Design review of the part built by this model. Coordinates are the model's own, in mm. Face numbers are marked on the shaded views. Coordinates: 2 decimals unless noted, no trailing zeros. Write each loop counter-clockwise with the first axis right and the second up, starting at its lowest first coordinate (ties: lowest second). Pieces come first, ordered by that corner, then holes.
Q1. For pin 1 Ø3 at (x, y) = (-7, 2.5) entering from +Z; pin 2 Ø4 at (x, z) = (1.5, -2.5) entering from -Y; pin 3 Ø4 at (x, y) = (14.5, 10.5) entering from +Z, all flat-tipped, find the tip position at first contact; note any pin that passes through.
Q2. The part is to be moulded in two halves that separate along X. For the marked faces 1, 2 and 3, say which applies: released by +X, released by -X, zero draft, split by the parting line, or undercut.
Q3. For L1, parallel to Y at x = 0, z = -3.5; L2, parallel to X at y = 2.25, z = 0.75; L3, parallel to X at y = 9.5, z = 0.25, list the stretches that pass through material, from the lowest coordinate up.
Q4. Take a section at B-B, the plane x = 28.5. Write out the cut boundary in (y, z).
Q5. Take a section at C-C, the plane z = 3.25. Write out the cut boundary in (x, y).
Q6. Take a section at D-D, the plane y = 11. Write out the cut boundary in (x, z), plus the area to 3 significant figures.
Q7. Take a section at A-A, the plane y = 6. Write out the cut boundary in (x, z), plus the area to 3 significant figures.
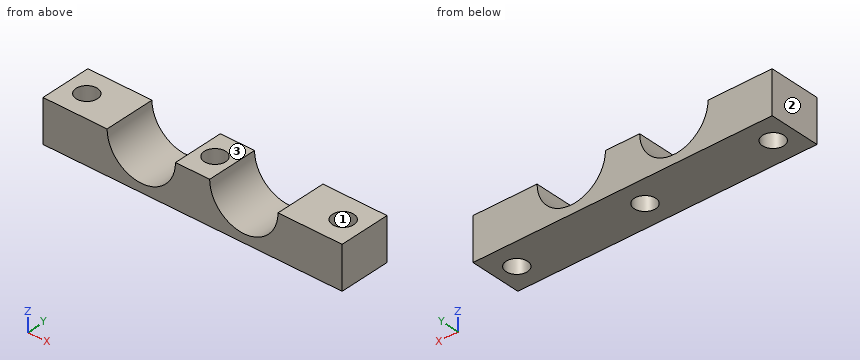
from build123d import *

# Parameters (mm, degrees)
BOSS_EXTRUDE1_DEPTH = 12
SKETCH2_R           = 2.5
CUT_EXTRUDE1_DEPTH  = 10


with BuildPart() as part:
    # Sketch1 → Boss-Extrude1 (new body)
    with BuildSketch(Plane(origin=(0, 0, 0), x_dir=(1, 0, 0), z_dir=(0, 1, 0))):
        with BuildLine():
            Line((35, 5), (-35, 5))
            Line((-35, 5), (-35, -5))
            Line((-35, -5), (-20, -5))
            ThreePointArc((-20, -5), (-12, 3), (-4, -5))
            Line((-4, -5), (4, -5))
            ThreePointArc((4, -5), (12, 3), (20, -5))
            Line((20, -5), (35, -5))
            Line((35, -5), (35, 5))
        make_face()
    extrude(amount=BOSS_EXTRUDE1_DEPTH)

    # Sketch2 → Cut-Extrude1 (cut)
    with BuildSketch(Plane(origin=(0, 0, -5), x_dir=(-1, 0, 0), z_dir=(0, 0, -1))):
        with Locations((0, 6)):
            Circle(SKETCH2_R)
        with Locations((-30, 6)):
            Circle(SKETCH2_R)
        with Locations((30, 6)):
            Circle(SKETCH2_R)
    extrude(amount=-CUT_EXTRUDE1_DEPTH, mode=Mode.SUBTRACT)


solid = part.part
Responses:
1. pin 1: stops at z = 0.34
1. pin 2: stops at y = 0
1. pin 3: stops at z = -1.61
2. face 1: undercut
2. face 2: released by -X
2. face 3: zero draft
3. L1: y = 0 to 3.5, 8.5 to 12
3. L2: x = -35 to -18.78, -5.22 to 5.22, 18.78 to 35
3. L3: x = -35 to -18.44, -5.56 to 5.56, 18.44 to 35
4. outline: (0, -5) - (4, -5) - (4, 5) - (0, 5) - close; (8, -5) - (12, -5) - (12, 5) - (8, 5) - close
5. outline: (-35, 0) - (-19.81, 0) - (-19.81, 12) - (-35, 12) - close; (-4.19, 0) - (4.19, 0) - (4.19, 12) - (-4.19, 12) - close; (19.81, 0) - (35, 0) - (35, 12) - (19.81, 12) - close; hole circle Ø5 at (-30, 6); hole circle Ø5 at (0, 6); hole circle Ø5 at (30, 6)
6. outline: (-35, -5) - (35, -5) - (35, 5) - (20, 5) arc R8 cw to (4, 5) - (-4, 5) arc R8 cw to (-20, 5) - (-35, 5) - close
6. area: 499 mm2
7. outline: (-35, -5) - (-32.5, -5) - (-32.5, 5) - (-35, 5) - close; (-27.5, -5) - (-2.5, -5) - (-2.5, 5) - (-4, 5) arc R8 cw to (-20, 5) - (-27.5, 5) - close; (2.5, -5) - (27.5, -5) - (27.5, 5) - (20, 5) arc R8 cw to (4, 5) - (2.5, 5) - close; (32.5, -5) - (35, -5) - (35, 5) - (32.5, 5) - close
7. area: 349 mm2
